Here's how the part is built. I have some questions about the finished solid (model axes, mm). A direction names the side the tool comes from. Round coordinates to 2 decimals unless told otherwise and drop trailing zeros. Loops run counter-clockwise (first coordinate to the right, second up) from the corner with the lowest first, then second, coordinate; pieces in that order, holes last. Notation, with made-up numbers: (66, 61.25) - (112, 61.25) arc R9 ccw to (112, 72.25) - close; hole circle Ø11 at (42, -34). An arc over 180 degrees is marked (long way). Return JSON: item names as keys, results as strings. Group by question number.
Autodesk Inventor part; units mm, degrees
ref_plane "YZ Plane" through (0, 0, 0) normal (1, 0, 0) x (0, 1, 0)
ref_plane "XZ Plane" through (0, 0, 0) normal (0, 1, 0) x (-1, 0, 0)
ref_plane "XY Plane" through (0, 0, 0) normal (0, 0, 1) x (1, 0, 0)
sketch "Sketch1" plane through (0, 0, 0) normal (0, 0, 1) x (1, 0, 0)
  line L0 (15, -15) -> (-15, -15)
  line L1 (-15, -15) -> (-15, 15)
  line L2 (-15, 15) -> (15, 15)
  line L3 (15, 15) -> (15, -15)
  line L4 (15, -15) -> (-15, 15) construction
  line L5 (-15, -15) -> (15, 15) construction
  point P0 (0, 0)
  dimension "d0" = 30
  dimension "d1" = 30
extrude "Extrusion1" add sketch "Sketch1" along normal blind 10
sketch "Sketch2" plane through (0, 0, 10) normal (0, 0, 1) x (1, 0, 0)
  circle A0 centre (0, 0) radius 7
  dimension "d4" = 14
extrude "Extrusion2" cut sketch "Sketch2" against normal blind 2
fillet "Fillet1" radius 2 8 edges at (0, 15, 10) (15, 0, 10) (15, 15, 5) (15, -15, 5) (0, -15, 10) (-15, -15, 5) (-15, 0, 10) (-15, 15, 5)
properties part number "potentiometer body"
Q1. If we mould it in two halves opening along Y, with no side actions, what happens to faces 3 (the cylindrical face through (-14.4, 14.43, 4.06)), 4 (the flat face through (0, 0, 8)), 5 (the cylindrical face through (-0.18, -14.43, 9.4))? For each: +Y half, -Y half, draft (parallel to the pull), parting line (faces both ways), or undercut.
Q2. Imagine slicing it at C-C, the plane z = 8.5. List the corners of the cut face in (x, y) for me, and give its area (3 significant figures).
Q3. Imagine slicing it at A-A, the plane x = 0. List the corners of the cut face in (y, z) for me, and give its area (3 significant figures).
Q4. For faces 1 (the cylindrical face through (6.466, -2.681, 9.014)), 2 (the cylindrical face through (14.4, -14.43, 4.06)), which set-ups out of +Z, -Z, +X, -X, +Y, -Y let a thin tool reach every point of the face, with its end or its side?
Q5. Please list where these lines run through material, in increasing order: line 1 (Y direction, x = 0, z = 9.25); line 2 (X direction, y = -2.5, z = 8.5); line 3 (Y direction, x = 0, z = 9.3).
Output values:
{
 "1": {"face 3": "+Y half", "face 4": "undercut", "face 5": "-Y half"},
 "2": {"outline": "(-14.94, -13) arc R1.94 ccw to (-13, -14.94) - (13, -14.94) arc R1.94 ccw to (14.94, -13) - (14.94, 13) arc R1.94 ccw to (13, 14.94) - (-13, 14.94) arc R1.94 ccw to (-14.94, 13) - close; hole circle Ø14 at (0, 0)", "area": "735 mm^2"},
 "3": {"outline": "(-15, 0) - (15, 0) - (15, 8) arc R2 ccw to (13, 10) - (7, 10) - (7, 8) - (-7, 8) - (-7, 10) - (-13, 10) arc R2 ccw to (-15, 8) - close", "area": "270 mm^2"},
 "4": {"face 1": "+Z", "face 2": "+Z, -Z, +X, -Y"},
 "5": {"line 1": "y = -14.56 to -7, 7 to 14.56", "line 2": "x = -14.94 to -6.54, 6.54 to 14.94", "line 3": "y = -14.52 to -7, 7 to 14.52"}
}
